Geometry: final body of the model. Coordinates: model frame, mm. Face numbers are marked on the shaded views. A direction names the side the tool comes from. Coordinates: 2 decimals unless noted, no trailing zeros. Loops run counter-clockwise (first coordinate to the right, second up) from the corner with the lowest first, then second, coordinate; pieces in that order, holes last. Notation, with made-up numbers: (13.25, 64) - (19.25, 64) arc R29 cw to (19.25, 94) - close; hole circle Ø3 at (71.25, -27). An arc over 180 degrees is marked (long way). Put each result on its own line as item: value. Start each with the question number.
1) Material intervals for line 1 along Y through (x, z) = (-30, 12); line 2 along X through (y, z) = (-39, 13); line 3 along X through (y, z) = (-59.25, 23.5), sorted ascending. Write a range as from..to.
2) Reachability of the marked faces 4 and 5 from +Z, -Z, +X, -X, +Y, -Y: full face, straight path, thin tool, end or side. Return the list, or none.
3) Contact query for flat-ended pins moving along their axis: pin 1 Ø4 at (y, z) = (-9, 20.5) entering from +X; pin 2 Ø10 at (x, y) = (15.5, -33) entering from +Z. Output: stop coordinate, or through.
4) Section A-A on x = -26. Output: boundary loops of the cut face in (y, z), and give its area (3 significant figures).
5) Section D-D on y = -34. Output: boundary loops of the cut face in (x, z).
6) Section B-B on y = -54.5. Output: boundary loops of the cut face in (x, z), and give its area (3 significant figures).
7) Section C-C on z = 34.5. Output: boundary loops of the cut face in (x, y).
8) Draft query along X for the marked faces 1, 2 and 3. Return one class per face: +X half, -X half, draft (parallel to the pull), parting line (faces both ways), or undercut.
```python
from build123d import *

# Parameters (mm, degrees)
SKETCH_1_W           = 99
SKETCH_1_H           = 104
SKETCH_1_R           = 1.5
SKETCH_1_W_2         = 95
SKETCH_1_H_2         = 61
EXTRUDE_3_DEPTH      = 3
SKETCH_3_W           = 99
SKETCH_3_H           = 104
SKETCH_3_W_2         = 95
SKETCH_3_H_2         = 100
EXTRUDE_4_DEPTH      = 33
CUT_EXTRUDE_2_DEPTH  = 30
SKETCH_5_W           = 50
SKETCH_5_H           = 7.5
CUT_EXTRUDE_3_DEPTH  = 30
SKETCH_6_W           = 28
SKETCH_6_H           = 55
CUT_EXTRUDE_4_DEPTH  = 30
SKETCH_7_W           = 7.5
SKETCH_7_H           = 18.5
CUT_EXTRUDE_5_DEPTH  = 30
SKETCH_8_W           = 25
SKETCH_8_H           = 7.5
CUT_EXTRUDE_6_DEPTH  = 30
FILLET_1_R           = 1
SKETCH_9_W           = 2
SKETCH_9_H           = 55
EXTRUDE_5_DEPTH      = 7.5
SKETCH_14_W          = 95
SKETCH_14_H          = 33
SKETCH_14_W_2        = 25
SKETCH_14_H_2        = 7.5
EXTRUDE_6_DEPTH      = 3
SKETCH_15_W          = 178.19226754
SKETCH_15_H          = 134.394802541
CUT_EXTRUDE_8_DEPTH  = 3
EXTRUDE_7_DEPTH      = 3
SKETCH_17_W          = 7.5
SKETCH_17_H          = 17
CUT_EXTRUDE_9_DEPTH  = 3
FILLET_3_R           = 1
SKETCH_19_W          = 95
SKETCH_19_H          = 97
EXTRUDE_8_DEPTH      = 2.5
SKETCH_20_W          = 2
SKETCH_20_H          = 20.5
EXTRUDE_9_DEPTH      = 2.5
CUT_EXTRUDE_10_DEPTH = 2
EXTRUDE_11_DEPTH     = 2
SKETCH_24_R          = 1.5
CUT_EXTRUDE_11_DEPTH = 2
SKETCH_25_R          = 1.5
CUT_EXTRUDE_12_DEPTH = 2
SKETCH_26_R          = 1.5
CUT_EXTRUDE_13_DEPTH = 2
SKETCH_27_R          = 1.5
CUT_EXTRUDE_14_DEPTH = 2
SKETCH_28_W          = 2
SKETCH_28_H          = 16.5
CUT_EXTRUDE_15_DEPTH = 4
SKETCH_29_W          = 6
SKETCH_29_H          = 7.5
EXTRUDE_12_DEPTH     = 2
SKETCH_30_W          = 6
SKETCH_30_H          = 7.5
CUT_EXTRUDE_16_DEPTH = 2


with BuildPart() as part:
    # 草图1 → 凸台-拉伸3 (new body)
    with BuildSketch(Plane.XY):
        with Locations((0, -11.5)):
            Rectangle(SKETCH_1_W, SKETCH_1_H)
        with Locations((43, 34)):
            Circle(SKETCH_1_R, mode=Mode.SUBTRACT)
        with Locations(Location((-43.5, 34, 0), (0, 0, 180))):
            Circle(SKETCH_1_R, mode=Mode.SUBTRACT)
        with Locations((-43.5, -34)):
            Circle(SKETCH_1_R, mode=Mode.SUBTRACT)
        with Locations(Location((43, -34, 0), (0, 0, 180))):
            Circle(SKETCH_1_R, mode=Mode.SUBTRACT)
        Rectangle(SKETCH_1_W_2, SKETCH_1_H_2, mode=Mode.SUBTRACT)
    extrude(amount=EXTRUDE_3_DEPTH)

    # 草图3 → 凸台-拉伸4 (add)
    with BuildSketch(Plane.XY.offset(3)):
        with Locations((0, -11.5)):
            Rectangle(SKETCH_3_W, SKETCH_3_H)
        with Locations((0, -11.5)):
            Rectangle(SKETCH_3_W_2, SKETCH_3_H_2, mode=Mode.SUBTRACT)
    extrude(amount=EXTRUDE_4_DEPTH)

    # 草图4 → 切除-拉伸2 (cut)
    with BuildSketch(Plane.ZY.offset(-47.5)):
        Polygon((12, 14.5), (12, -30.5), (3, -30.5), (0, -30.5), (0, 14.5), align=None)
    extrude(amount=-CUT_EXTRUDE_2_DEPTH, mode=Mode.SUBTRACT)

    # 草图5 → 切除-拉伸3 (cut)
    with BuildSketch(Plane(origin=(0, 40.5, 0), x_dir=(1, 0, 0), z_dir=(0, 1, 0))):
        with Locations((-10, -24.75)):
            Rectangle(SKETCH_5_W, SKETCH_5_H)
    extrude(amount=-CUT_EXTRUDE_3_DEPTH, mode=Mode.SUBTRACT)

    # 草图6 → 切除-拉伸4 (cut)
    with BuildSketch(Plane.ZY.offset(-47.5)):
        with Locations((22, 11)):
            Rectangle(SKETCH_6_W, SKETCH_6_H)
    extrude(amount=-CUT_EXTRUDE_4_DEPTH, mode=Mode.SUBTRACT)

    # 草图7 → 切除-拉伸5 (cut)
    with BuildSketch(Plane.ZY.offset(-47.5)):
        with Locations((27.75, -39.75)):
            Rectangle(SKETCH_7_W, SKETCH_7_H)
    extrude(amount=-CUT_EXTRUDE_5_DEPTH, mode=Mode.SUBTRACT)

    # 草图8 → 切除-拉伸6 (cut)
    with BuildSketch(Plane(origin=(0, -61.5, 0), x_dir=(1, 0, 0), z_dir=(0, 1, 0))):
        with Locations((27.5, -24.75)):
            Rectangle(SKETCH_8_W, SKETCH_8_H)
    extrude(amount=-CUT_EXTRUDE_6_DEPTH, mode=Mode.SUBTRACT)

    # 圆角1
    fillet_1_edges = [part.edges().sort_by_distance(p)[0] for p in [
        (-49.5, 40.5, 18),
        (49.5, 40.5, 18),
        (49.5, -63.5, 18),
        (-49.5, -63.5, 18),
    ]]
    fillet(fillet_1_edges, radius=FILLET_1_R)

    # 草图9 → 凸台-拉伸5 (add)
    with BuildSketch(Plane.XY.offset(36)):
        with Locations((48.5, 11)):
            Rectangle(SKETCH_9_W, SKETCH_9_H)
    extrude(amount=-EXTRUDE_5_DEPTH)

    # 草图14 → 凸台-拉伸6 (add)
    with BuildSketch(Plane(origin=(0, -61.5, 0), x_dir=(1, 0, 0), z_dir=(0, 1, 0))):
        with Locations((0, -19.5)):
            Rectangle(SKETCH_14_W, SKETCH_14_H)
        with Locations((27.5, -24.75)):
            Rectangle(SKETCH_14_W_2, SKETCH_14_H_2, mode=Mode.SUBTRACT)
    extrude(amount=EXTRUDE_6_DEPTH)

    # 草图15 → 切除-拉伸8 (cut)
    with BuildSketch(Plane.XZ.offset(63.5)):
        with Locations((3.050514682, 15.901855456)):
            Rectangle(SKETCH_15_W, SKETCH_15_H)
    extrude(amount=-CUT_EXTRUDE_8_DEPTH, mode=Mode.SUBTRACT)

    # 草图16 → 凸台-拉伸7 (add)
    with BuildSketch(Plane(origin=(0, 0, 0), x_dir=(-1, 0, 0), z_dir=(0, 0, -1))):
        Polygon((-47.5, 30.5), (-46.5, 30.5), (-46.5, -30.5), (-49.5, -30.5), (-49.5, 14.5), (-47.5, 14.5), align=None)
    extrude(amount=-EXTRUDE_7_DEPTH)

    # 草图17 → 切除-拉伸9 (cut)
    with BuildSketch(Plane.ZY.offset(49.5)):
        with Locations((24.25, -37.5)):
            Rectangle(SKETCH_17_W, SKETCH_17_H)
    extrude(amount=-CUT_EXTRUDE_9_DEPTH, mode=Mode.SUBTRACT)

    # 圆角3
    fillet_3_edges = [part.edges().sort_by_distance(p)[0] for p in [
        (49.5, -60.5, 18),
        (-49.5, -60.5, 18),
    ]]
    fillet(fillet_3_edges, radius=FILLET_3_R)

    # 草图19 → 凸台-拉伸8 (add)
    with BuildSketch(Plane.XY.offset(36)):
        with BuildLine():
            Line((-49.5, 39.5), (-49.5, -59.5))
            ThreePointArc((-49.5, -59.5), (-49.207106781, -60.207106781), (-48.5, -60.5))
            Line((-48.5, -60.5), (48.5, -60.5))
            ThreePointArc((48.5, -60.5), (49.207106781, -60.207106781), (49.5, -59.5))
            Line((49.5, -59.5), (49.5, 39.5))
            ThreePointArc((49.5, 39.5), (49.207106781, 40.207106781), (48.5, 40.5))
            Line((48.5, 40.5), (-48.5, 40.5))
            ThreePointArc((-48.5, 40.5), (-49.207106781, 40.207106781), (-49.5, 39.5))
        make_face()
        with Locations((0, -10)):
            Rectangle(SKETCH_19_W, SKETCH_19_H, mode=Mode.SUBTRACT)
    extrude(amount=EXTRUDE_8_DEPTH)

    # 草图20 → 凸台-拉伸9 (add)
    with BuildSketch(Plane.XZ.offset(-38.5)):
        with Locations((48.5, 18.25)):
            Rectangle(SKETCH_20_W, SKETCH_20_H)
    extrude(amount=EXTRUDE_9_DEPTH)

    # 草图21 → 切除-拉伸10 (cut)
    with BuildSketch(Plane.XZ.offset(60.5)):
        Polygon((43, 24), (43, 31.5), (18, 31.5), (18, 28.5), (40, 28.5), (40, 24), align=None)
    extrude(amount=-CUT_EXTRUDE_10_DEPTH, mode=Mode.SUBTRACT)

    # 草图23 → 凸台-拉伸11 (add)
    with BuildSketch(Plane.XZ.offset(60.5)):
        Polygon((15, 28.5), (18, 28.5), (18, 24), (40, 24), (40, 21), (15, 21), align=None)
    extrude(amount=-EXTRUDE_11_DEPTH)

    # 草图24 → 切除-拉伸11 (cut)
    with BuildSketch(Plane(origin=(49.5, 0, 0), x_dir=(0, 0, -1), z_dir=(1, 0, 0))):
        with Locations((-23.5, -54.5)):
            Circle(SKETCH_24_R)
    extrude(amount=-CUT_EXTRUDE_11_DEPTH, mode=Mode.SUBTRACT)

    # 草图25 → 切除-拉伸12 (cut)
    with BuildSketch(Plane.XZ.offset(60.5)):
        with Locations(Location((-41.5, 23.5, 0), (0, 0, 270))):
            Circle(SKETCH_25_R)
    extrude(amount=-CUT_EXTRUDE_12_DEPTH, mode=Mode.SUBTRACT)

    # 草图26 → 切除-拉伸13 (cut)
    with BuildSketch(Plane.ZY.offset(49.5)):
        with Locations((23.5, 33.5)):
            Circle(SKETCH_26_R)
    extrude(amount=-CUT_EXTRUDE_13_DEPTH, mode=Mode.SUBTRACT)

    # 草图27 → 切除-拉伸14 (cut)
    with BuildSketch(Plane(origin=(0, 40.5, 0), x_dir=(1, 0, 0), z_dir=(0, 1, 0))):
        with Locations(Location((42.5, -23.5, 0), (0, 0, 270))):
            Circle(SKETCH_27_R)
    extrude(amount=-CUT_EXTRUDE_14_DEPTH, mode=Mode.SUBTRACT)

    # 草图28 → 切除-拉伸15 (cut)
    with BuildSketch(Plane(origin=(0, -16.5, 0), x_dir=(1, 0, 0), z_dir=(0, 1, 0))):
        with Locations((48.5, -20.25)):
            Rectangle(SKETCH_28_W, SKETCH_28_H)
    extrude(amount=-CUT_EXTRUDE_15_DEPTH, mode=Mode.SUBTRACT)

    # 草图29 → 凸台-拉伸12 (add)
    with BuildSketch(Plane.XZ.offset(60.5)):
        with Locations((40, 27.75)):
            Rectangle(SKETCH_29_W, SKETCH_29_H)
    extrude(amount=-EXTRUDE_12_DEPTH)

    # 草图30 → 切除-拉伸16 (cut)
    with BuildSketch(Plane.XZ.offset(60.5)):
        with Locations((15, 27.75)):
            Rectangle(SKETCH_30_W, SKETCH_30_H)
    extrude(amount=-CUT_EXTRUDE_16_DEPTH, mode=Mode.SUBTRACT)


solid = part.part
```
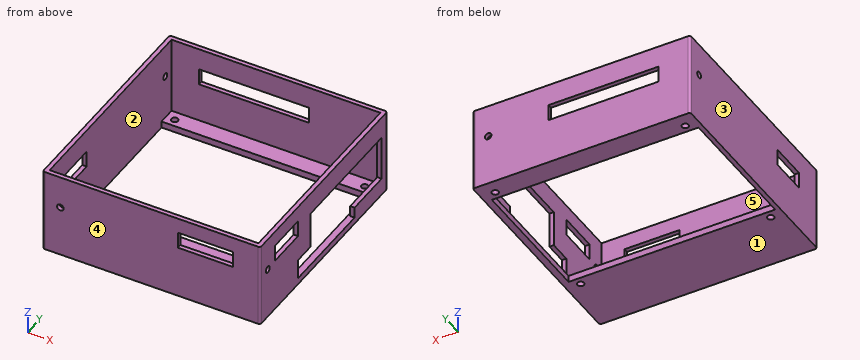
Answer block:
1. line 1: y = -60.5..-58.5, 38.5..40.5
1. line 2: x = -49.5..-47.5, 47.5..49.5
1. line 3: x = -49.5..-43, -40..49.5
2. face 4: +Z, -Z, +X, -X, -Y
2. face 5: +Z
3. pin 1: stops at x = -47.5
3. pin 2: stops at z = 3
4. outline: (-60.5, 0) - (-30.5, 0) - (-30.5, 3) - (-58.5, 3) - (-58.5, 38.5) - (-60.5, 38.5) - close; (30.5, 0) - (40.5, 0) - (40.5, 21) - (38.5, 21) - (38.5, 3) - (30.5, 3) - close; (38.5, 28.5) - (40.5, 28.5) - (40.5, 38.5) - (38.5, 38.5) - close
4. area: 247 mm²
5. outline: (-49.5, 0) - (-45, 0) - (-45, 3) - (-47.5, 3) - (-47.5, 20.5) - (-49.5, 20.5) - close; (-49.5, 28) - (-47.5, 28) - (-47.5, 38.5) - (-49.5, 38.5) - close; (-42, 0) - (41.5, 0) - (41.5, 3) - (-42, 3) - close; (44.5, 0) - (49.5, 0) - (49.5, 24) - (47.5, 24) - (47.5, 3) - (44.5, 3) - close; (47.5, 31.5) - (49.5, 31.5) - (49.5, 38.5) - (47.5, 38.5) - close
6. outline: (-49.5, 0) - (49.5, 0) - (49.5, 22) - (47.5, 22) - (47.5, 3) - (-47.5, 3) - (-47.5, 38.5) - (-49.5, 38.5) - close; (47.5, 25) - (49.5, 25) - (49.5, 38.5) - (47.5, 38.5) - close
6. area: 433 mm²
7. outline: (-49.5, -59.5) arc R1 ccw to (-48.5, -60.5) - (48.5, -60.5) arc R1 ccw to (49.5, -59.5) - (49.5, 39.5) arc R1 ccw to (48.5, 40.5) - (-48.5, 40.5) arc R1 ccw to (-49.5, 39.5) - close; hole (-47.5, -58.5) - (47.5, -58.5) - (47.5, 38.5) - (-47.5, 38.5) - close
8. face 1: draft
8. face 2: undercut
8. face 3: -X half
